Answer from the drawing. Dimensions are ordinates in mm from the lowest x, y and z of the part. A direction names the side the tool comes from. Coordinates: 2 decimals unless noted, no trailing zeros. Loops run counter-clockwise (first coordinate to the right, second up) from the corner with the lowest first, then second, coordinate; pieces in that order, holes last. Notation, with made-up numbers: M 10,73.25 L 54,73.25 A19 cw 54,78.25 Z; hole C -14.75,-12.5 d7. An arc over 180 degrees is marked long. Put each result on its own line as item: value.
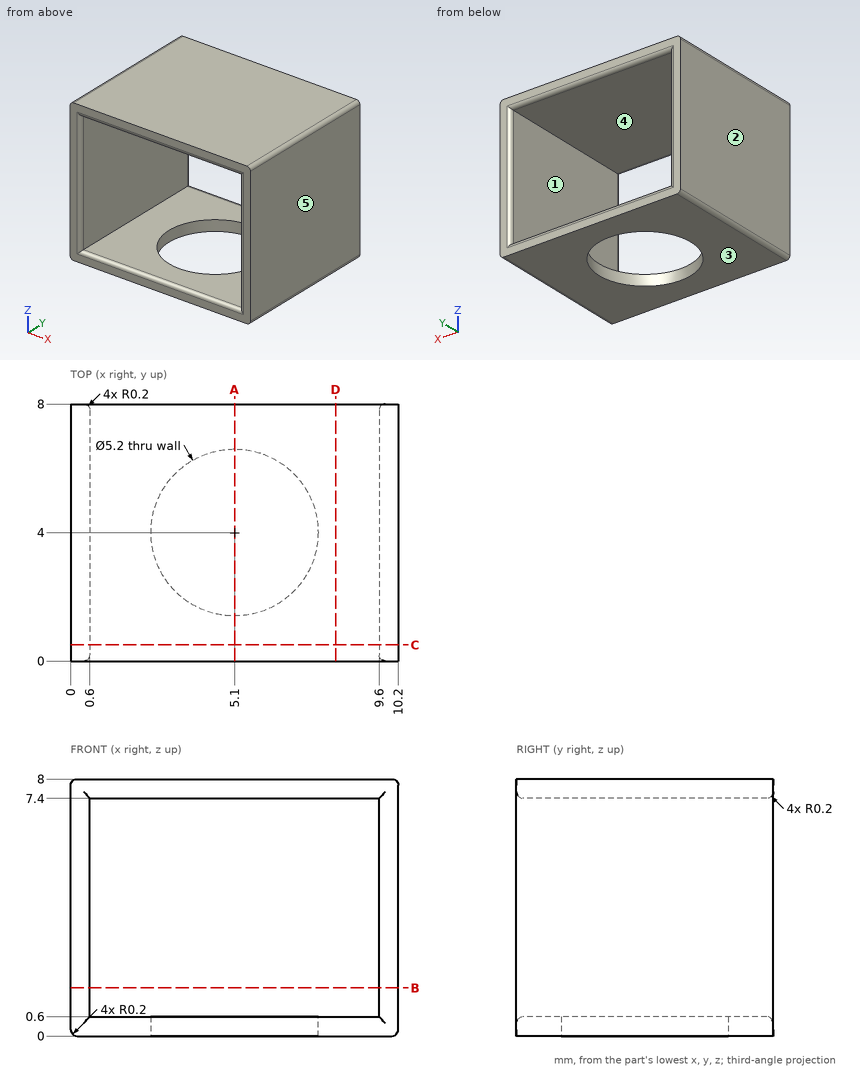
1) Find section C-C, the plane y = 0.5. Write down the section's boundary in (x, z), plus the area to 3 significant figures.
Answer list:
outline: M 0,0.2 A0.2 ccw 0.2,0 L 10,0 A0.2 ccw 10.2,0.2 L 10.2,7.8 A0.2 ccw 10,8 L 0.2,8 A0.2 ccw 0,7.8 Z; hole M 0.6,0.6 L 9.6,0.6 L 9.6,7.4 L 0.6,7.4 Z
area: 20.4 mm^2
2) Find section B-B, the plane z = 1.5. Write down the section's boundary in (x, y).
Answer list:
outline: M 0,0 L 0.4,0 A0.2 ccw 0.6,0.2 L 0.6,7.8 A0.2 ccw 0.4,8 L 0,8 Z; M 9.6,0.2 A0.2 ccw 9.8,0 L 10.2,0 L 10.2,8 L 9.8,8 A0.2 ccw 9.6,7.8 Z
3) Find section D-D, the plane x = 8.25. Write down the section's boundary in (y, z), plus the area to 3 significant figures.
Answer list:
outline: M 0,0 L 8,0 L 8,0.4 A0.2 ccw 7.8,0.6 L 0.2,0.6 A0.2 ccw 0,0.4 Z; M 0,7.6 A0.2 ccw 0.2,7.4 L 7.8,7.4 A0.2 ccw 8,7.6 L 8,8 L 0,8 Z
area: 9.57 mm^2
4) Which of the six approach directions +Z, -Z, +X, -X, +Y, -Y give full straight-line access (tool end or side, diameter ignored) to the marked faces 4 and 5?
Answer list:
face 4: +Y, -Y
face 5: +Z, -Z, +X, +Y, -Y
5) Determine the mould class of the marked faces 1, 2 and 3 for opening direction X: released by +X, released by -X, zero draft, split by the parting line, or undercut.
Answer list:
face 1: undercut
face 2: released by -X
face 3: zero draft
6) Straight lines are drawn through the part: line 1 (Y direction, x = 5.1, z = 0.3); line 2 (Z direction, x = 1, y = 6); line 3 (X direction, y = 4, z = 0.25). For each, find the intervals that lie inside material, in ascending order. Write a range as [from, to].
Answer list:
line 1: y = [0, 1.4], [6.6, 8]
line 2: z = [0, 0.6], [7.4, 8]
line 3: x = [0, 2.5], [7.7, 10.2]
7) Find section A-A, the plane x = 5.1. Write down the section's boundary in (y, z).
Answer list:
outline: M 0,0 L 1.4,0 L 1.4,0.6 L 0.2,0.6 A0.2 ccw 0,0.4 Z; M 0,7.6 A0.2 ccw 0.2,7.4 L 7.8,7.4 A0.2 ccw 8,7.6 L 8,8 L 0,8 Z; M 6.6,0 L 8,0 L 8,0.4 A0.2 ccw 7.8,0.6 L 6.6,0.6 Z
